The listing builds one solid part. Answer for the finished solid, in the listing's coordinates (mm). Round coordinates to 2 decimals unless told otherwise and drop trailing zeros. Write each loop counter-clockwise with the first axis right and the second up, starting at its lowest first coordinate (ties: lowest second). Pieces come first, ordered by that corner, then holes. Notation, with made-up numbers: (25, -6.5) - (79, -6.5) arc R8 cw to (79, 1.5) - close; hole circle Ø5 at (55.25, 21.25). An arc over 180 degrees is marked (long way). Return JSON: item names as keys, results as strings. Group by question number.
(1) Section B-B, the plane y = 0 is taken. Write down the section's boundary in (x, z).
(2) Section C-C, the plane z = 20.5 is taken. Write down the section's boundary in (x, y).
(3) Section D-D, the plane z = 110 is taken. Write down the section's boundary in (x, y).
(4) Each of these flat-tipped pins is pushed along its axis until it touches: pin 1 (1 mm diameter, centred on y = 4.5, z = 25, fed in from -X); pin 2 (8 mm diameter, centred on x = 8.5, z = 110, fed in from +Y); pin 3 (1 mm diameter, centred on x = 5.5, z = 102, fed in from +Y). Where does it stop, or does it pass through?
(5) Find the intervals of material crossed by line 1 along X through (y, z) = (5, 158); line 2 along Y through (x, z) = (9.5, 128); line 3 along Y through (x, z) = (-0.5, 55), in increasing order. Write a range as [from, to].
(6) Section A-A, the plane x = 0 is taken. Write down the section's boundary in (y, z), then the cut area to 3 significant figures.
```python
from build123d import *

# Parameters (mm, degrees)
SKETCH1_R               = 17.78
BOSS_EXTRUDE1_DEPTH     = 111.76
SKETCH2_R               = 12.7
BOSS_EXTRUDE2_DEPTH     = 63.5
BOSS_EXTRUDE2_TAPER     = 7
CUT_EXTRUDE1_DEPTH      = 178.054580285
CUT_EXTRUDE1_DEPTH_BACK = 178.054580285


with BuildPart() as part:
    # Sketch1 → Boss-Extrude1 (new body)
    with BuildSketch(Plane.XY):
        Circle(SKETCH1_R)
    extrude(amount=BOSS_EXTRUDE1_DEPTH)

    # Sketch2 → Boss-Extrude2 (add)
    with BuildSketch(Plane.XY.offset(111.76)):
        Circle(SKETCH2_R)
    extrude(amount=BOSS_EXTRUDE2_DEPTH, taper=BOSS_EXTRUDE2_TAPER)

    # Sketch4 → Cut-Extrude1 (cut, two sides: drawn at the far end of the back side and taken through both)
    with BuildSketch(Plane(origin=(0, 0, 0), x_dir=(0, 0, -1), z_dir=(1, 0, 0)).offset(-CUT_EXTRUDE1_DEPTH_BACK)):
        Polygon((16.51, 49.579194367), (-26.426841821, -24.789597184), (59.446841821, -24.789597184), align=None)
    extrude(amount=CUT_EXTRUDE1_DEPTH + CUT_EXTRUDE1_DEPTH_BACK, mode=Mode.SUBTRACT)


solid = part.part
```
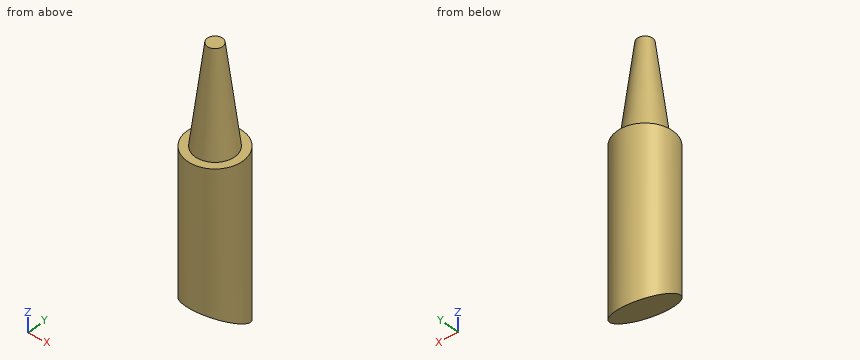
Working result:
{
 "1": {"outline": "(-17.78, 12.11) - (17.78, 12.11) - (17.78, 111.76) - (12.7, 111.76) - (4.9, 175.26) - (-4.9, 175.26) - (-12.7, 111.76) - (-17.78, 111.76) - close"},
 "2": {"outline": "(-10.26, -14.52) - (10.26, -14.52) arc R17.78 ccw (long way) to start"},
 "3": {"outline": "circle Ø35.56 at (0, 0)"},
 "4": {"pin 1": "stops at x = -17.32", "pin 2": "stops at y = 17.2", "pin 3": "stops at y = 17.06"},
 "5": {"line 1": "x = [-4.93, 4.93]", "line 2": "y = [-4.94, 4.94]", "line 3": "y = [-17.77, 17.77]"},
 "6": {"outline": "(-17.78, 22.38) - (17.78, 1.85) - (17.78, 111.76) - (12.7, 111.76) - (4.9, 175.26) - (-4.9, 175.26) - (-12.7, 111.76) - (-17.78, 111.76) - close", "area": "4,660 mm^2"}
}
